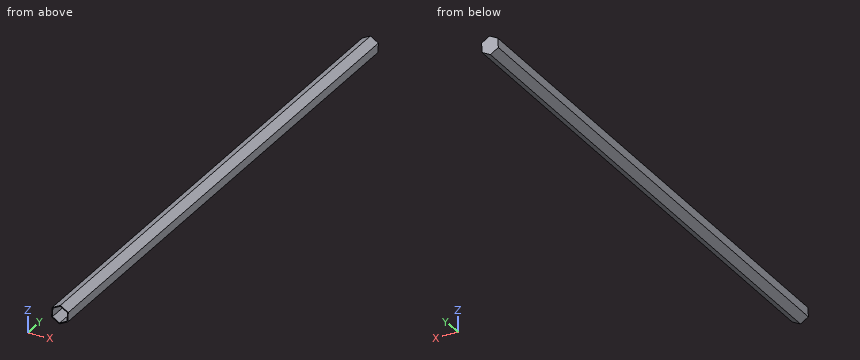
```python
from build123d import *

# Parameters (mm, degrees)
F1_DEPTH = 1752.6
F2_T     = -2.54


with BuildPart() as f1:
    # F0 (on Front) → F1 (new body)
    with BuildSketch(Plane.XZ):
        Polygon((-1.279764, -29.30146), (24.735926, -15.759038), (26.01569, 13.542422), (1.279764, 29.30146), (-24.735926, 15.759038), (-26.01569, -13.542422), align=None)
    extrude(amount=-F1_DEPTH)

    # F2
    f2_openings = [f1.faces().sort_by_distance(p)[0] for p in [
        (0, 0, 0),
    ]]
    offset(amount=F2_T, openings=f2_openings)


solid = f1.part
```
Design review of the part built by this model. Coordinates are the model's own, in mm. Round coordinates to 2 decimals unless told otherwise and drop trailing zeros. Write each loop counter-clockwise with the first axis right and the second up, starting at its lowest first coordinate (ties: lowest second). Pieces come first, ordered by that corner, then holes.
Item 1: We need section C-C on z = -1. Write out the cut boundary in (x, y), and give its area (3 significant figures).
Item 2: We need section A-A on y = 109. Write out the cut boundary in (x, z), and give its area (3 significant figures).
Item 3: We need section B-B on x = 13. Write out the cut boundary in (y, z), and give its area (3 significant figures).
Item 4: Clearance check with flat-ended pins moving along their axes: pin 1 Ø3 at (x, z) = (20, 1) entering from -Y; pin 2 Ø8 at (x, y) = (-18.5, 1132) entering from -Z; pin 3 Ø10 at (y, z) = (231, -18.5) entering from +X. State where each tip first meets the part, or that it passes through.
Item 5: For probe 1 along X at (y, z) = (805.5, -8.5); probe 2 along X at (y, z) = (812.5, -13); probe 3 along Z at (x, y) = (-12, 212.5), list the stretches that pass through material, from the lowest coordinate up.
Returned:
1. outline: (-25.47, 0) - (-22.93, 0) - (-22.93, 1750.06) - (22.84, 1750.06) - (22.84, 0) - (25.38, 0) - (25.38, 1752.6) - (-25.47, 1752.6) - close
1. area: 9,030 mm2
2. outline: (-26.02, -13.54) - (-1.28, -29.3) - (24.74, -15.76) - (26.02, 13.54) - (1.28, 29.3) - (-24.74, 15.76) - close; hole (-23.41, -12.19) - (-1.15, -26.37) - (22.26, -14.18) - (23.41, 12.19) - (1.15, 26.37) - (-22.26, 14.18) - close
2. area: 425 mm2
3. outline: (0, -21.87) - (1752.6, -21.87) - (1752.6, 21.83) - (0, 21.83) - (0, 18.82) - (1750.06, 18.82) - (1750.06, -19) - (0, -19) - close
3. area: 10,400 mm2
4. pin 1: stops at y = 1750.06
4. pin 2: stops at z = -20.88
4. pin 3: stops at x = 24.83
5. probe 1: x = -25.8 to -23.25, 22.51 to 25.05
5. probe 2: x = -25.99 to -22.14, 22.31 to 24.86
5. probe 3: z = -22.47 to -19.46, 19.53 to 22.39
